Geometry: final body of the model. Coordinates: model frame, mm. Face numbers are marked on the shaded views. A direction names the side the tool comes from. Give positions to 0.01 mm unless a question says otherwise; leave off trailing zeros. Write each loop counter-clockwise with the first axis right and the second up, starting at its lowest first coordinate (ties: lowest second). Pieces come first, ordered by that corner, then holes. Notation, with made-up numbers: M 16.25,50 L 70.25,50 A25 ccw 70.25,69 Z; hole C 22,-5.5 d3. An arc over 180 degrees is marked long. Answer as a JSON object with one key per item and string values.
from build123d import *

# Parameters (mm, degrees)
CYLINDER013_R     = 1
CYLINDER013_DEPTH = 10
CYLINDER014_R     = 1
CYLINDER014_DEPTH = 10
CYLINDER017_R     = 1
CYLINDER017_DEPTH = 10
CYLINDER011_R     = 1
CYLINDER011_DEPTH = 10
BOX001_W          = 10
BOX001_H          = 40
BOX001_DEPTH      = 70
CYLINDER016_R     = 3
CYLINDER016_DEPTH = 10
CYLINDER015_R     = 3
CYLINDER015_DEPTH = 10
CYLINDER012_R     = 3
CYLINDER012_DEPTH = 10
CYLINDER010_R     = 3
CYLINDER010_DEPTH = 10
BOX_W             = 10
BOX_H             = 40
BOX_DEPTH         = 70
BOX002_W          = 45
BOX002_H          = 40
BOX002_DEPTH      = 10
FILLET_R          = 6


with BuildPart() as foro001:
    # Cylinder013 → Cylinder013 (new body)
    with BuildSketch(Plane(origin=(47, 36.5, 48), x_dir=(0, 0, -1), z_dir=(1, 0, 0))):
        Circle(CYLINDER013_R)
    extrude(amount=CYLINDER013_DEPTH)


with BuildPart() as foro002:
    # Cylinder014 → Cylinder014 (new body)
    with BuildSketch(Plane(origin=(22, 36.5, 62), x_dir=(1, 0, 0), z_dir=(0, 0, 1))):
        Circle(CYLINDER014_R)
    extrude(amount=CYLINDER014_DEPTH)


with BuildPart() as foro003:
    # Cylinder017 → Cylinder017 (new body)
    with BuildSketch(Plane(origin=(22, 3.5, 62), x_dir=(1, 0, 0), z_dir=(0, 0, 1))):
        Circle(CYLINDER017_R)
    extrude(amount=CYLINDER017_DEPTH)


with BuildPart() as foro:
    # Cylinder011 → Cylinder011 (new body)
    with BuildSketch(Plane(origin=(47, 3.5, 48), x_dir=(0, 0, -1), z_dir=(1, 0, 0))):
        Circle(CYLINDER011_R)
    extrude(amount=CYLINDER011_DEPTH)


with BuildPart() as cube001:
    # Box001 → Box001 (new body)
    with BuildSketch(Plane(origin=(45, 0, 0), x_dir=(1, 0, 0), z_dir=(0, 0, 1))):
        with Locations((5, 20)):
            Rectangle(BOX001_W, BOX001_H)
    extrude(amount=BOX001_DEPTH)


with BuildPart() as cylinder016:
    # Cylinder016 → Cylinder016 (new body)
    with BuildSketch(Plane(origin=(22, 3.5, 62), x_dir=(1, 0, 0), z_dir=(0, 0, 1))):
        Circle(CYLINDER016_R)
    extrude(amount=CYLINDER016_DEPTH)


with BuildPart() as cylinder015:
    # Cylinder015 → Cylinder015 (new body)
    with BuildSketch(Plane(origin=(22, 36.5, 62), x_dir=(1, 0, 0), z_dir=(0, 0, 1))):
        Circle(CYLINDER015_R)
    extrude(amount=CYLINDER015_DEPTH)


with BuildPart() as cylinder012:
    # Cylinder012 → Cylinder012 (new body)
    with BuildSketch(Plane(origin=(47, 36.5, 48), x_dir=(0, 0, -1), z_dir=(1, 0, 0))):
        Circle(CYLINDER012_R)
    extrude(amount=CYLINDER012_DEPTH)


with BuildPart() as cylinder010:
    # Cylinder010 → Cylinder010 (new body)
    with BuildSketch(Plane(origin=(47, 3.5, 48), x_dir=(0, 0, -1), z_dir=(1, 0, 0))):
        Circle(CYLINDER010_R)
    extrude(amount=CYLINDER010_DEPTH)


with BuildPart() as cube:
    # Box → Box (new body)
    with BuildSketch(Plane(origin=(-10, 0, 0), x_dir=(1, 0, 0), z_dir=(0, 0, 1))):
        with Locations((5, 20)):
            Rectangle(BOX_W, BOX_H)
    extrude(amount=BOX_DEPTH)


with BuildPart() as fillet_body:
    # Box002 → Box002 (new body)
    with BuildSketch(Plane.XY.offset(60)):
        with Locations((22.5, 20)):
            Rectangle(BOX002_W, BOX002_H)
    extrude(amount=BOX002_DEPTH)

    # Fusion: union Cube001, Cylinder016, Cylinder015, Cylinder012, Cylinder010, Cube
    add(cube001.part)
    add(cylinder016.part)
    add(cylinder015.part)
    add(cylinder012.part)
    add(cylinder010.part)
    add(cube.part)

    # Cut: cut foro
    add(foro.part, mode=Mode.SUBTRACT)

    # Cut001: cut foro003
    add(foro003.part, mode=Mode.SUBTRACT)

    # Cut002: cut foro002
    add(foro002.part, mode=Mode.SUBTRACT)

    # Cut003: cut foro001
    add(foro001.part, mode=Mode.SUBTRACT)

    # Fillet
    fillet_edges = [fillet_body.edges().sort_by_distance(p)[0] for p in [
        (50, 0, 0),
        (-5, 0, 0),
        (50, 40, 0),
        (55, 20, 0),
        (55, 20, 70),
        (-10, 20, 70),
        (-10, 20, 0),
        (-5, 40, 0),
    ]]
    fillet(fillet_edges, radius=FILLET_R)


solid = fillet_body.part
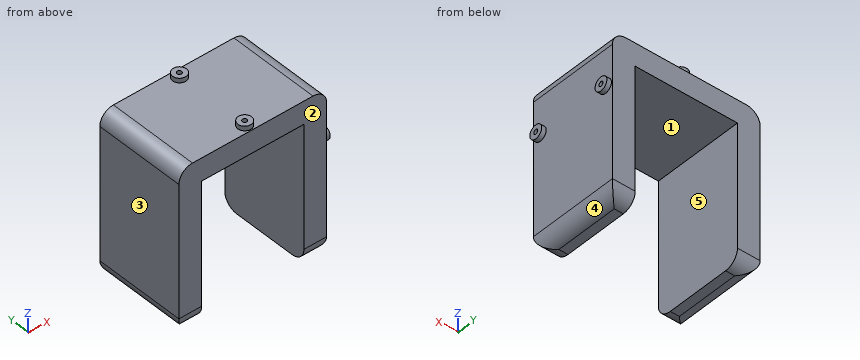
1) Cut plane A-A on z = 23.5. Return loops of the section in (x, y).
Geometry check:
{"outline": "M -10,0 L 0,0 L 0,40 L -10,40 Z; M 45,0 L 55,0 L 55,40 L 45,40 Z"}
2) Cut plane C-C on x = 22. Return loops of the section in (y, z), and give its area (3 significant figures).
Geometry check:
{"outline": "M 0,60 L 40,60 L 40,70 L 39.5,70 L 39.5,72 L 37.5,72 L 37.5,62 L 35.5,62 L 35.5,72 L 33.5,72 L 33.5,70 L 6.5,70 L 6.5,72 L 4.5,72 L 4.5,62 L 2.5,62 L 2.5,72 L 0.5,72 L 0.5,70 L 0,70 Z", "area": "384 mm2"}
3) Cut plane D-D on z = 48. Return loops of the section in (x, y), and give its area (3 significant figures).
Geometry check:
{"outline": "M -10,0 L 0,0 L 0,40 L -10,40 Z; M 45,0 L 55,0 L 55,0.5 L 57,0.5 L 57,2.5 L 47,2.5 L 47,4.5 L 57,4.5 L 57,6.5 L 55,6.5 L 55,33.5 L 57,33.5 L 57,35.5 L 47,35.5 L 47,37.5 L 57,37.5 L 57,39.5 L 55,39.5 L 55,40 L 45,40 Z", "area": "784 mm2"}
4) Set-up query: the marked faces 1 and 2. Return all of +Z, -Z, +X, -X, +Y, -Y with unobstructed straight access to the full face (end or side cutting, diameter ignored); none if empty.
Geometry check:
{"face 1": "-Z, +Y, -Y", "face 2": "+Z, -Z, +X, -X, -Y"}
5) Cut plane B-B on y = 20.5. Return loops of the section in (x, z), and give its area (3 significant figures).
Geometry check:
{"outline": "M -10,6 A6 ccw -4,0 L 0,0 L 0,60 L 45,60 L 45,0 L 49,0 A6 ccw 55,6 L 55,64 A6 ccw 49,70 L -4,70 A6 ccw -10,64 Z", "area": "1,820 mm2"}
6) Contact query for flat-ended pins moving along their axis: P1, Ø20, axis at y = 14, z = 25, coming from the +X side; P2, Ø2.5, axis at x = 22, y = 3.5, coming from the -Z side; P3, Ø20, axis at x = 35, y = 17.5, coming from the +Z side; P4, Ø1, axis at y = 3, z = 48.5, coming from the +X side. Output: stop coordinate, or through.
Geometry check:
{"P1": "stops at x = 55", "P2": "stops at z = 60", "P3": "stops at z = 70", "P4": "stops at x = 57"}
7) Pull-direction query (X, two-part tool) for the marked faces 3, 4 and 5; classes: pulls with the +X half, pulls with the -X half, needs draft (parallel to the pull), parting line crosses it, or undercut.
Geometry check:
{"face 3": "pulls with the -X half", "face 4": "pulls with the +X half", "face 5": "undercut"}
8) Line query: line 1 (Y direction, x = 51, z = 48); line 2 (X direction, y = 20.5, z = 17.5); line 3 (Z direction, x = 42, y = 27). Output: solid intervals per line, ascending. Write a range as from..to.
Geometry check:
{"line 1": "y = 0..2.5, 4.5..35.5, 37.5..40", "line 2": "x = -10..0, 45..55", "line 3": "z = 60..70"}
